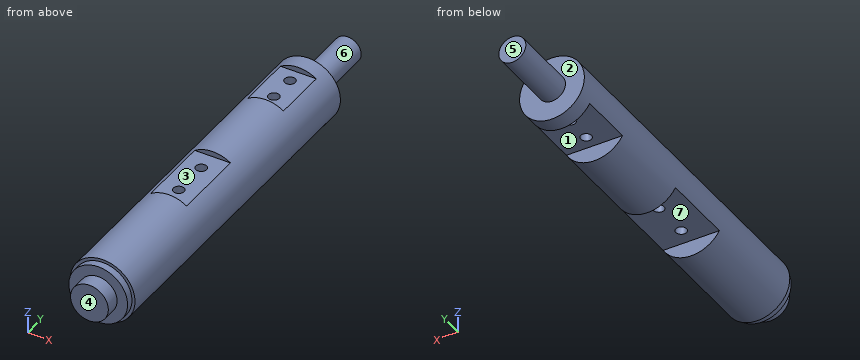
from build123d import *

# Parameters (mm, degrees)
SKETCH1_R               = 19.05
BOSS_EXTRUDE1_DEPTH     = 254
SKETCH2_W               = 11.1125
SKETCH2_H               = 38.989
CUT_EXTRUDE1_DEPTH      = 256.424754086
CUT_EXTRUDE1_DEPTH_BACK = 256.424754086
SKETCH3_W               = 9.525
SKETCH3_H               = 32.258
SKETCH3_H_2             = 43.18
SKETCH3_W_2             = 3.175
F_1_1_DIAMETER_HOLE1_D  = 6.35


with BuildPart() as part:
    # Sketch1 → Boss-Extrude1 (new body)
    with BuildSketch(Plane(origin=(0, 0, 0), x_dir=(1, 0, 0), z_dir=(0, 1, 0))):
        with Locations(Location((0, 0, 0), (0, 0, 270))):
            Circle(SKETCH1_R)
    extrude(amount=BOSS_EXTRUDE1_DEPTH)

    # Sketch2 → Cut-Revolve1 (revolve, cut)
    with BuildSketch(Plane.XY, mode=Mode.PRIVATE) as cut_revolve1_sk:
        Polygon((19.05, 0), (11.1125, 0), (11.1125, 8.636), (17.272, 8.636), (17.272, 12.954), (19.05, 12.954), align=None)
        with Locations((13.49375, 234.5055)):
            Rectangle(SKETCH2_W, SKETCH2_H)
    revolve(cut_revolve1_sk.sketch.rotate(Axis((0, 348.337253792, 0), (0, -1, 0)), 90), axis=Axis((0, 348.337253792, 0), (0, -1, 0)), mode=Mode.SUBTRACT)

    # Sketch3 → Cut-Extrude1 (cut, two sides: drawn at the far end of the back side and taken through both)
    with BuildSketch(Plane(origin=(0, 0, 0), x_dir=(0, 0, -1), z_dir=(1, 0, 0)).offset(-CUT_EXTRUDE1_DEPTH_BACK)):
        with Locations((14.2875, 189.357)):
            Rectangle(SKETCH3_W, SKETCH3_H)
        with Locations((14.2875, 99.568)):
            Rectangle(SKETCH3_W, SKETCH3_H_2)
        with Locations((-17.4625, 189.357)):
            Rectangle(SKETCH3_W_2, SKETCH3_H)
        with Locations((-17.4625, 99.568)):
            Rectangle(SKETCH3_W_2, SKETCH3_H_2)
    extrude(amount=CUT_EXTRUDE1_DEPTH + CUT_EXTRUDE1_DEPTH_BACK, mode=Mode.SUBTRACT)

    # 1 (1) Diameter Hole1 (through all)
    with Locations(Plane(origin=(0, 0, -9.525), x_dir=(-1, 0, 0), z_dir=(0, 0, -1))):
        with Locations((0, 197.2945), (0, 181.4195), (0, 109.982), (0, 87.884)):
            Hole(F_1_1_DIAMETER_HOLE1_D / 2)


solid = part.part
Verification items for the finished model (mm, model axes). Face numbers are marked on the shaded views. A direction names the side the tool comes from. Coordinates: 2 decimals unless noted, no trailing zeros. Order: outer loops, then holes, each group sorted by start corner. A loop starts at its lowest first (then second) coordinate and runs counter-clockwise, first axis right, second up. Notation, with made-up numbers: (66.5, 81) -> (86.5, 81) arc R21 ccw to (86.5, 101) -> close; hole circle Ø7 at (53.5, 21). An arc over 180 degrees is marked (long way). Use CSV: the item, a comma, the result in double quotes. Start each with the question number.
Q1. Depth check by flat-ended pin: P1, Ø1, axis at x = -2, z = 13, coming from the -Y side; P2, Ø1.6, axis at x = -1.5, z = 18, coming from the +Y side; P3, Ø16.5, axis at x = -3.5, y = 110, coming from the -Z side (3 decimals). Enter the tip coordinate at first touch or a pass-through.
Q2. Section check A-A, the plane z = 0. Give the number of separate pieces and of enclosed holes in the cut face, and give its area (3 significant figures).
Q3. Section check D-D, the plane y = 80.5. Record the cut outline in (x, z) (3 decimals), and give its area (3 significant figures).
Q4. Thickness scan on line 1 along Y through (x, z) = (14.5, -11); line 2 along Y through (x, z) = (-2.5, -12.5); line 3 along Y through (x, z) = (0, -2). Record the ranges inside material, lowest first.
Q5. Section check C-C, the plane y = 171. Record the cut outline in (x, z).
Q6. Tool access check on the marked faces 1, 2 and 3. Record the directions out of +Z, -Z, +X, -X, +Y, -Y that give a thin tool (end or side, any length) a straight path to the whole face; none if there is none.
Q7. Draft check along Y on the marked faces 4, 5, 6 and 7. Enter one of: +Y half, -Y half, draft (parallel to the pull), parting line (faces both ways), or undercut.
Returned:
1,P1,"stops at y = 8.64"
1,P2,"stops at y = 215.01"
1,P3,"stops at z = -9.525"
2,separate pieces,"1"
2,enclosed holes,"4"
2,area,"8,530 mm^2"
3,outline,"(-16.498, -9.525) -> (16.498, -9.525) arc R19.05 ccw to (10.53, 15.875) -> (-10.53, 15.875) arc R19.05 ccw to start"
3,area,"872 mm^2"
4,line 1,"y = 12.95 to 77.98, 121.16 to 173.23, 205.49 to 215.01"
4,line 2,"y = 8.64 to 77.98, 121.16 to 173.23, 205.49 to 215.01"
4,line 3,"y = 0 to 84.71, 91.06 to 106.81, 113.16 to 178.24, 184.59 to 194.12, 200.47 to 254"
5,outline,"circle Ø38.1 at (0, 0)"
6,face 1,"-Z, +X, -X"
6,face 2,"+Y"
6,face 3,"+Z, +X, -X"
7,face 4,"-Y half"
7,face 5,"+Y half"
7,face 6,"draft"
7,face 7,"undercut"
